Input: part model. Units: mm. Frame: model coordinates. A direction names the side the tool comes from. Give positions to 0.01 mm unless a question says otherwise; leave off trailing zeros. Loops run counter-clockwise (first coordinate to the right, second up) from the corner with the lowest first, then second, coordinate; pieces in that order, holes last. Notation, with made-up numbers: M 88.25,-20.5 L 94.25,-20.5 A13 ccw 94.25,-4.5 Z; hole C 81,73 d6. An arc over 180 degrees is marked long. One line per item, written item: value. Start each with the question number.
(1) Pull-direction query (X, two-part tool) for faces 1 (the flat face through (12.68, -0.41, -16.49)), 2 (the flat face through (15.12, -2, -12)), 3 (the conical face through (-13.92, -0.32, -20.76)); classes: released by +X, released by -X, zero draft, split by the parting line, or undercut.
(2) Pin query (flat end, axial travel): P1, Ø5, axis at x = -8, z = 8, coming from the -Y side; P2, Ø1.5, axis at y = -1.5, z = 15.5, coming from the -X side; P3, Ø3, axis at x = -10.18, z = -14.86, coming from the -Y side; P4, Ø1.6, axis at y = -1, z = 14, coming from the +X side. Return the tip coordinate at first contact, or that it passes through.
(3) Access query for faces 4 (the flat face through (-9.668, -0.406, -19.58)), 5 (the flat face through (0, -1, 18.88)), 6 (the flat face through (0, -2, 9)). Directions: +Z, -Z, +X, -X, +Y, -Y. A direction counts if a zero-diameter tool reaches every point of the face in a straight line with its end or side. Return the directions, or none.
(4) Section B-B on z = 12. Output: boundary loops of the cut face in (x, y), plus the area to 3 significant figures.
(5) Ray query, line 1 along Y through (x, z) = (7, 16); line 2 along X through (y, z) = (-1.55, -17); line 3 along Z through (x, y) = (7, -2.6). Return the intervals inside material, ascending. Write a range as from..to.
(6) Section A-A on x = 3. Output: boundary loops of the cut face in (y, z), plus the area to 3 significant figures.
```python
from build123d import *

# Parameters (mm, degrees)
PAD013_DEPTH    = 2
PAD014_DEPTH    = 1.2
POCKET011_DEPTH = 3.201
CHAMFER010_SIZE = 0.8


with BuildPart() as part:
    # Sketch034 → Pad013 (new body)
    with BuildSketch(Plane.XZ):
        with BuildLine():
            ThreePointArc((-7.12, 25), (-9.24132, 24.12132), (-10.12, 22))
            Line((-10.12, 22), (-10.12, 2))
            Line((-10.12, 2), (-12.12, -2))
            ThreePointArc((-12.12, -2), (-14.24132, -2.87868), (-15.12, -5))
            Line((-15.12, -5), (-15.12, -19))
            ThreePointArc((-15.12, -19), (-14.24132, -21.12132), (-12.12, -22))
            Line((-12.12, -22), (12.12, -22))
            ThreePointArc((12.12, -22), (14.24132, -21.12132), (15.12, -19))
            Line((15.12, -19), (15.12, -5))
            ThreePointArc((15.12, -5), (14.24132, -2.87868), (12.12, -2))
            Line((10.12, 2), (12.12, -2))
            Line((10.12, 22), (10.12, 2))
            ThreePointArc((10.12, 22), (9.24132, 24.12132), (7.12, 25))
            Line((-7.12, 25), (7.12, 25))
        make_face()
        with BuildLine():
            Line((-3.5, 18.88), (3.5, 18.88))
            ThreePointArc((4, 18.38), (3.853553, 18.733553), (3.5, 18.88))
            Line((4, 18.38), (4, 11.38))
            ThreePointArc((3.5, 10.88), (3.853553, 11.026447), (4, 11.38))
            Line((3.5, 10.88), (-3.5, 10.88))
            ThreePointArc((-4, 11.38), (-3.853553, 11.026447), (-3.5, 10.88))
            Line((-4, 11.38), (-4, 18.38))
            ThreePointArc((-3.5, 18.88), (-3.853553, 18.733553), (-4, 18.38))
        make_face(mode=Mode.SUBTRACT)
    extrude(amount=PAD013_DEPTH)

    # Sketch035 → Pad014 (join)
    with BuildSketch(Plane.XZ.offset(2)):
        with BuildLine():
            ThreePointArc((15.12, -5), (14.24132, -2.87868), (12.12, -2))
            Line((-12.12, -2), (12.12, -2))
            ThreePointArc((-12.12, -2), (-14.24132, -2.87868), (-15.12, -5))
            Line((-15.12, -19), (-15.12, -5))
            ThreePointArc((-15.12, -19), (-14.24132, -21.12132), (-12.12, -22))
            Line((12.12, -22), (-12.12, -22))
            ThreePointArc((12.12, -22), (14.24132, -21.12132), (15.12, -19))
            Line((15.12, -5), (15.12, -19))
        make_face()
    extrude(amount=PAD014_DEPTH)

    # Sketch062 → Pocket011 (cut, through all)
    with BuildSketch(Plane.XZ):
        with BuildLine():
            ThreePointArc((-12.892741, -18.792945), (-12.685685, -19.565685), (-11.912945, -19.772741))
            Line((-11.912945, -19.772741), (-7.566279, -18.608055))
            ThreePointArc((-7.566279, -18.608055), (-6.511508, -16.428232), (-8.82149, -15.70149))
            ThreePointArc((-8.82149, -15.70149), (-9.548232, -13.391508), (-11.728055, -14.446279))
            Line((-12.892741, -18.792945), (-11.728055, -14.446279))
        make_face()
        with BuildLine():
            ThreePointArc((11.912945, -19.772741), (12.685685, -19.565685), (12.892741, -18.792945))
            Line((12.892741, -18.792945), (11.728055, -14.446279))
            ThreePointArc((11.728055, -14.446279), (9.548232, -13.391508), (8.82149, -15.70149))
            ThreePointArc((8.82149, -15.70149), (6.511508, -16.428232), (7.566279, -18.608055))
            Line((11.912945, -19.772741), (7.566279, -18.608055))
        make_face()
    extrude(amount=POCKET011_DEPTH, mode=Mode.SUBTRACT)

    # Chamfer010
    chamfer010_edges = [part.edges().sort_by_distance(p)[0] for p in [
        (-12.685685, 0, -19.565685),
        (-11.912945, -1.6, -19.772741),
        (-12.685685, -3.2, -19.565685),
        (-12.892741, -1.6, -18.792945),
        (9.739612, 0, -19.190398),
        (7.566279, -1.6, -18.608055),
        (9.739612, -3.2, -19.190398),
        (11.912945, -1.6, -19.772741),
        (0, 0, -22),
        (-14.24132, -3.2, -21.12132),
    ]]
    chamfer(chamfer010_edges, length=CHAMFER010_SIZE)


solid = part.part
```
Output values:
1. face 1: undercut
1. face 2: released by +X
1. face 3: released by -X
2. P1: stops at y = -2
2. P2: stops at x = -10.12
2. P3: passes through
2. P4: stops at x = 10.12
3. face 4: +Y
3. face 5: +Y, -Y
3. face 6: +Z, +X, -X, -Y
4. outline: M -10.12,-2 L -4,-2 L -4,0 L -10.12,0 Z; M 4,-2 L 10.12,-2 L 10.12,0 L 4,0 Z
4. area: 24.5 mm²
5. line 1: y = -2..0
5. line 2: x = -15.12..-12.41, -6.38..6.38, 12.41..15.12
5. line 3: z = -21.8..-18.57, -15.55..-2.2
6. outline: M -3.2,-21.2 L -2.4,-22 L -0.8,-22 L 0,-21.2 L 0,10.88 L -2,10.88 L -2,-2 L -2.4,-2 L -3.2,-2.8 Z; M -2,18.88 L 0,18.88 L 0,25 L -2,25 Z
6. area: 101 mm²
